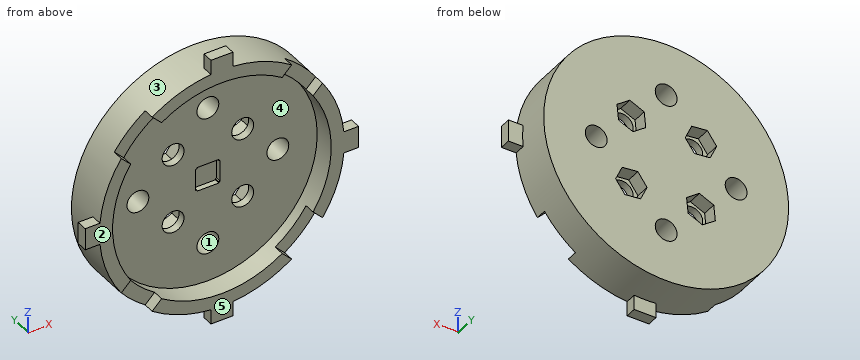
from build123d import *

# Parameters (mm, degrees)
BOSS_EXTRUDE1_DEPTH      = 15
BOSS_EXTRUDE1_DEPTH_BACK = 5
SKETCH1_R                = 56
SKETCH1_R_2              = 5
BOSS_EXTRUDE3_DEPTH      = 5
SKETCH4_R                = 50
CUT_EXTRUDE1_DEPTH       = 10
CUT_EXTRUDE2_DEPTH       = 5
CUT_EXTRUDE5_START       = -10
CUT_EXTRUDE5_DEPTH       = 2.5
CUT_EXTRUDE6_DEPTH       = 6.5


with BuildPart() as part:
    # Sketch1 → Boss-Extrude1 (new, two sides: drawn at the far end of the back side and taken through both)
    with BuildSketch(Plane(origin=(0, 0, 0), x_dir=(1, 0, 0), z_dir=(0, 1, 0)).offset(-BOSS_EXTRUDE1_DEPTH_BACK)):
        with Locations(Location((0, 0, 0), (0, 0, 270))):
            Circle(SKETCH1_R)
        with Locations(Location((15.909902577, 15.909902577, 0), (0, 0, 270))):
            Circle(SKETCH1_R_2, mode=Mode.SUBTRACT)
        with Locations(Location((15.909902577, -15.909902577, 0), (0, 0, 270))):
            Circle(SKETCH1_R_2, mode=Mode.SUBTRACT)
        with Locations(Location((-15.909902577, -15.909902577, 0), (0, 0, 270))):
            Circle(SKETCH1_R_2, mode=Mode.SUBTRACT)
        with Locations(Location((-15.909902577, 15.909902577, 0), (0, 0, 270))):
            Circle(SKETCH1_R_2, mode=Mode.SUBTRACT)
        with Locations(Location((-32, 0, 0), (0, 0, 270))):
            Circle(SKETCH1_R_2, mode=Mode.SUBTRACT)
        with Locations(Location((0, 32, 0), (0, 0, 270))):
            Circle(SKETCH1_R_2, mode=Mode.SUBTRACT)
        with Locations(Location((32, 0, 0), (0, 0, 270))):
            Circle(SKETCH1_R_2, mode=Mode.SUBTRACT)
        with Locations(Location((0, -32, 0), (0, 0, 270))):
            Circle(SKETCH1_R_2, mode=Mode.SUBTRACT)
    extrude(amount=BOSS_EXTRUDE1_DEPTH + BOSS_EXTRUDE1_DEPTH_BACK)

    # Sketch3 → Boss-Extrude3 (add)
    with BuildSketch(Plane.XZ.offset(5)):
        Polygon((-5, 5), (-5, 62.5), (5, 62.5), (5, 5), (62.5, 5), (62.5, -5), (5, -5), (5, -62.5), (-5, -62.5), (-5, -5), (-62.5, -5), (-62.5, 5), align=None)
    extrude(amount=-BOSS_EXTRUDE3_DEPTH)

    # Sketch4 → Cut-Extrude1 (cut)
    with BuildSketch(Plane.XZ.offset(5)):
        with Locations(Location((0, 0, 0), (0, 0, 270))):
            Circle(SKETCH4_R)
    extrude(amount=-CUT_EXTRUDE1_DEPTH, mode=Mode.SUBTRACT)

    # Sketch5 → Cut-Extrude2 (cut)
    with BuildSketch(Plane.XZ.offset(5)):
        with BuildLine():
            Line((27.56994834, 41.712083963), (31.890451666, 46.032587289))
            ThreePointArc((31.890451666, 46.032587289), (39.597979746, 39.597979746), (46.032587289, 31.890451666))
            Line((46.032587289, 31.890451666), (41.712083963, 27.56994834))
            ThreePointArc((41.712083963, 27.56994834), (35.355339059, 35.355339059), (27.56994834, 41.712083963))
        make_face()
        with BuildLine():
            Line((41.712083963, -27.56994834), (46.032587289, -31.890451666))
            ThreePointArc((46.032587289, -31.890451666), (39.597979746, -39.597979746), (31.890451666, -46.032587289))
            Line((31.890451666, -46.032587289), (27.56994834, -41.712083963))
            ThreePointArc((27.56994834, -41.712083963), (35.355339059, -35.355339059), (41.712083963, -27.56994834))
        make_face()
        with BuildLine():
            Line((-27.56994834, -41.712083963), (-31.890451666, -46.032587289))
            ThreePointArc((-31.890451666, -46.032587289), (-39.597979746, -39.597979746), (-46.032587289, -31.890451666))
            Line((-46.032587289, -31.890451666), (-41.712083963, -27.56994834))
            ThreePointArc((-41.712083963, -27.56994834), (-35.355339059, -35.355339059), (-27.56994834, -41.712083963))
        make_face()
        with BuildLine():
            Line((-41.712083963, 27.56994834), (-46.032587289, 31.890451666))
            ThreePointArc((-46.032587289, 31.890451666), (-39.597979746, 39.597979746), (-31.890451666, 46.032587289))
            Line((-31.890451666, 46.032587289), (-27.56994834, 41.712083963))
            ThreePointArc((-27.56994834, 41.712083963), (-35.355339059, 35.355339059), (-41.712083963, 27.56994834))
        make_face()
    extrude(amount=-CUT_EXTRUDE2_DEPTH, mode=Mode.SUBTRACT)

    # Sketch8 → Cut-Extrude5 (cut)
    with BuildSketch(Plane(origin=(0, 15, 0), x_dir=(1, 0, 0), z_dir=(0, 1, 0)).offset(CUT_EXTRUDE5_START)):
        Polygon((-5, 5), (-5.590169944, 5), (-5.590169944, -5), (-5, -5), (-5, -5.590169944), (5, -5.590169944), (5, -5), (5.590169944, -5), (5.590169944, 5), (5, 5), (5, 5.590169944), (-5, 5.590169944), align=None)
    extrude(amount=CUT_EXTRUDE5_DEPTH, mode=Mode.SUBTRACT)

    # Sketch10 → Cut-Extrude6 (cut)
    with BuildSketch(Plane(origin=(0, 15, 0), x_dir=(1, 0, 0), z_dir=(0, 1, 0))):
        Polygon((11.688650249, 21.770596118), (8.723766922, 15.184537596), (12.94501925, 9.323844055), (20.131154904, 10.049209035), (23.096038231, 16.635267557), (18.874785904, 22.495961099), align=None)
        Polygon((-16.635267557, 23.096038231), (-22.495961099, 18.874785904), (-21.770596118, 11.688650249), (-15.184537596, 8.723766922), (-9.323844055, 12.94501925), (-10.049209035, 20.131154904), align=None)
        Polygon((21.770596118, -11.688650249), (15.184537596, -8.723766922), (9.323844055, -12.94501925), (10.049209035, -20.131154904), (16.635267557, -23.096038231), (22.495961099, -18.874785904), align=None)
        Polygon((-11.688650249, -21.770596118), (-8.723766922, -15.184537596), (-12.94501925, -9.323844055), (-20.131154904, -10.049209035), (-23.096038231, -16.635267557), (-18.874785904, -22.495961099), align=None)
    extrude(amount=-CUT_EXTRUDE6_DEPTH, mode=Mode.SUBTRACT)


solid = part.part
Model file for the job. Use its own axes, mm. Face numbers are marked on the shaded views. A direction names the side the tool comes from. Give positions to 0.01 mm unless a question says otherwise; leave off trailing zeros. Write each loop counter-clockwise with the first axis right and the second up, starting at its lowest first coordinate (ties: lowest second). Pieces come first, ordered by that corner, then holes. Notation, with made-up numbers: (76, -18.5) - (111, -18.5) arc R27 ccw to (111, 2.5) - close; hole circle Ø1 at (43, 36). An arc over 180 degrees is marked (long way). Answer as CSV lines item,"result".
1. Band-saw the part on B-B (z = 0). Write the cut outline in (x, y).
Responses:
outline,"(-62.5, -5) - (-50, -5) - (-50, 5) - (-37, 5) - (-37, 15) - (-56, 15) - (-56, 0) - (-62.5, 0) - close; (-27, 5) - (-5.59, 5) - (-5.59, 7.5) - (5.59, 7.5) - (5.59, 5) - (27, 5) - (27, 15) - (-27, 15) - close; (37, 5) - (50, 5) - (50, -5) - (62.5, -5) - (62.5, 0) - (56, 0) - (56, 15) - (37, 15) - close"
2. Two-plate mould, pull along Z, no slides. Class the marked faces 1, 2 and 3: +Z half, -Z half, draft (parallel to the pull), parting line (faces both ways), or undercut.
Responses:
face 1,"undercut"
face 2,"draft"
face 3,"parting line"
3. Band-saw the part on C-C (y = 13.5). Count the separate pieces of the cut face and the enclosed holes in it, and give its area (3 significant figures).
Responses:
separate pieces,"1"
enclosed holes,"8"
area,"9,000 mm2"
4. 3-axis set-ups, long thin cutter, end or side, ignore diameter. For the marked faces 4 and 5: which of +Z, -Z, +X, -X, +Y, -Y reach the whole face in a straight line?
Responses:
face 4,"-Y"
face 5,"+Z, -Z, +X, -X, -Y"
5. Band-saw the part on A-A (x = 0). Write the cut outline in (y, z).
Responses:
outline,"(-5, -62.5) - (0, -62.5) - (0, -56) - (15, -56) - (15, -37) - (5, -37) - (5, -50) - (-5, -50) - close; (-5, 50) - (5, 50) - (5, 37) - (15, 37) - (15, 56) - (0, 56) - (0, 62.5) - (-5, 62.5) - close; (5, -27) - (15, -27) - (15, 27) - (5, 27) - (5, 5.59) - (7.5, 5.59) - (7.5, -5.59) - (5, -5.59) - close"
6. Drill centre lines: L1, parallel to Z at x = -1, y = -2.25; L2, parallel to Z at x = 1.5, y = 6; L3, parallel to Y at x = -30.5, z = 34. Where is each one in solid material? Low to high. Write a range as [from, to].
Responses:
L1,"z = [-62.5, -49.99], [49.99, 62.5]"
L2,"z = [-55.98, -36.77], [-27.23, -5.59], [5.59, 27.23], [36.77, 55.98]"
L3,"y = [5, 15]"
7. Pin check, flat tips, straight feed: pin 1 (13 mm diameter, centred on x = 0, z = -32, fed in from -Y); pin 2 (4 mm diameter, centred on x = -39, z = 44.5, fed in from +Y); pin 3 (5.5 mm diameter, centred on x = 60.5, z = -2.5, fed in from +Y); pin 4 (0.6 mm diameter, centred on y = 6, z = -5.5, fed in from -X). Stop position of each tip, or through.
Responses:
pin 1,"stops at y = 5"
pin 2,"passes through"
pin 3,"stops at y = 0"
pin 4,"stops at x = -55.76"
